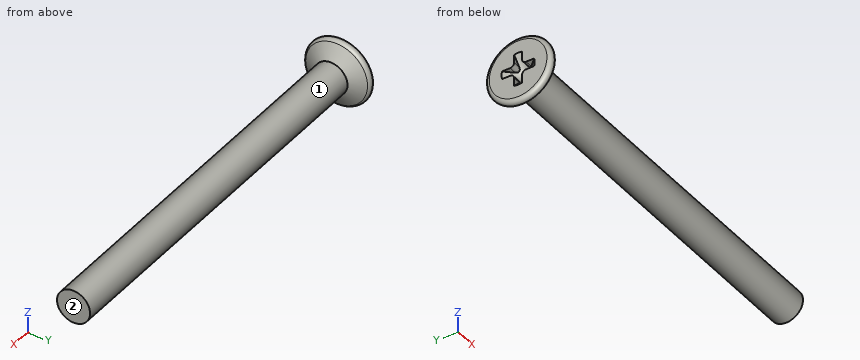
from build123d import *

# Parameters (mm, degrees)
RESSALTO_EXTRUS_O1_DEPTH = 1
PADR_OCIRCULAR1_COUNT    = 4


with BuildPart() as part:
    # Esboço1 → Revolução1 (revolve)
    with BuildSketch(Plane(origin=(0, 0, 0), x_dir=(1, 0, 0), z_dir=(0, 1, 0))):
        with BuildLine():
            Line((1.221687836, 1.25), (30, 1.25))
            Line((30, 1.25), (30, 0))
            Line((30, 0), (1.25, 0))
            Line((1.25, 0), (0, 1.25))
            Line((0, 1.25), (0, 2.183012702))
            ThreePointArc((0, 2.183012702), (0.234944948, 2.48919892), (0.591506351, 2.341506351))
            Line((0.591506351, 2.341506351), (1.221687836, 1.25))
        make_face()
    revolve(axis=Axis((0, 0, 0), (-1, 0, 0)))

    # Esboço2 → Ressalto-extrusão1 (add)
    with BuildSketch(Plane(origin=(0, 0, 0), x_dir=(0, 0, -1), z_dir=(1, 0, 0))):
        with BuildLine():
            Line((-0.3, 1.21346611), (-0.3, 0.6))
            ThreePointArc((-0.3, 0.6), (-0.387867966, 0.387867966), (-0.6, 0.3))
            Line((-0.6, 0.3), (-1.21346611, 0.3))
            ThreePointArc((-1.21346611, 0.3), (-0.924029762, 0.924029762), (-0.3, 1.21346611))
        make_face()
    ressalto_extrus_o1 = extrude(amount=RESSALTO_EXTRUS_O1_DEPTH)

    # PadrãoCircular1: Ressalto-extrusão1 ×4 about axis
    padr_ocircular1_axis = Axis((0, 0, 0), (1, 0, 0))
    for i in range(1, PADR_OCIRCULAR1_COUNT):
        add(ressalto_extrus_o1.rotate(padr_ocircular1_axis, i * 360 / PADR_OCIRCULAR1_COUNT))


solid = part.part
Could you check a few things on this model? Use its own coordinates, in mm. Face numbers are marked on the shaded views. A direction names the side the tool comes from. Round coordinates to 2 decimals unless told otherwise and drop trailing zeros. Loops run counter-clockwise (first coordinate to the right, second up) from the corner with the lowest first, then second, coordinate; pieces in that order, holes last. Notation, with made-up numbers: (5.5, 0.25) -> (58.5, 0.25) arc R18 cw to (58.5, 30.25) -> close; hole circle Ø9 at (89.5, 68.5). An arc over 180 degrees is marked (long way). Use CSV: the item, a comma, the result in double quotes.
(1) For the marked faces 1 and 2, which set-ups out of +Z, -Z, +X, -X, +Y, -Y let a thin tool reach every point of the face, with its end or its side?
Return value:
face 1,"+X"
face 2,"+Z, -Z, +X, +Y, -Y"
(2) Will these pins go through, and if not, where does the flat tip stop? pin 1 Ø0.5 at (x, z) = (0.5, 1) entering from -Y; pin 2 Ø0.6 at (x, z) = (0.5, 1) entering from +Y; pin 3 Ø0.6 at (x, y) = (0, 1) entering from -Z.
Return value:
pin 1,"stops at y = -2.37"
pin 2,"stops at y = 2.39"
pin 3,"stops at z = -2.35"
(3) Suppose I cut it at A-A on x = 4. Write out the boundary of the cut face in (y, z).
Return value:
outline,"circle Ø2.5 at (0, 0)"
(4) If I drill on probe 1 along Z at (x, y) = (29, -0.05); probe 2 along Y at (x, z) = (25, -0.3); probe 3 along X at (y, z) = (0.55, -1.2), over which ranges is the centre line in solid material (lowest first)? Write a range as [from, to].
Return value:
probe 1,"z = [-1.25, 1.25]"
probe 2,"y = [-1.21, 1.21]"
probe 3,"x = [0, 1.18]"
